Answer from the drawing. Dimensions are ordinates in mm from the lowest x, y and z of the part. A direction names the side the tool comes from. Give positions to 0.01 mm unless a question says otherwise; leave off trailing zeros. Loops run counter-clockwise (first coordinate to the right, second up) from the corner with the lowest first, then second, coordinate; pieces in that order, holes last. Notation, with made-up numbers: (72, 23) - (101, 23) arc R36 cw to (101, 60) - close; hole circle Ø9 at (65.25, 29.5). An arc over 180 degrees is marked (long way). One line per question, with ' | ' between items. Start each with the question number.
1. Which of the six approach directions +Z, -Z, +X, -X, +Y, -Y give full straight-line access (tool end or side, diameter ignored) to the marked faces 3 and 4?
2. Section C-C (z = 2.1) is taken. Determine the outline of the cut face in (x, y).
3. For a pull along Y with two mould halves and no side action, classify the marked faces 1 and 2 as released by +Y, released by -Y, zero draft, split by the parting line, or undercut.
4. Section A-A (y = 6.4) is taken. Determine the outline of the cut face in (x, z), plus the area to 3 significant figures.
5. Find the intervals of material crossed by line 1 (Y direction, x = 6.4, z = 0.35); line 2 (Y direction, x = 6.4, z = 1.85); line 3 (X direction, y = 6, z = 0.75), in increasing order.
6. Section D-D (z = 1.05) is taken. Determine the outline of the cut face in (x, y), plus the area to 3 significant figures.
7. Each of these flat-tipped pins is pushed along its axis until it touches: pin 1 (1 mm diameter, centred on x = 11.5, z = 1.5, fed in from +Y); pin 2 (1.4 mm diameter, centred on x = 6.4, y = 6.4, fed in from -Z). Where does it stop, or does it pass through?
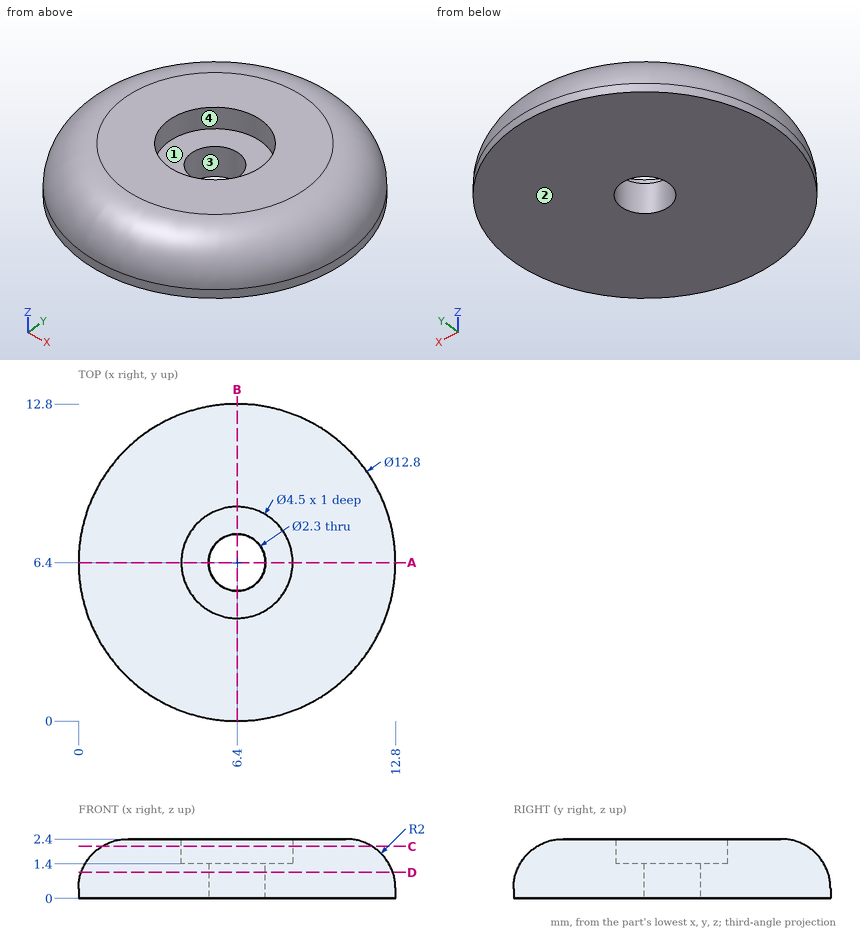
Conclusion:
1) face 3: +Z, -Z | face 4: +Z
2) outline: circle Ø10.91 at (6.4, 6.4); hole circle Ø4.5 at (6.4, 6.4)
3) face 1: undercut | face 2: zero draft
4) outline: (0, 0) - (5.25, 0) - (5.25, 1.4) - (4.15, 1.4) - (4.15, 2.4) - (2, 2.4) arc R2 ccw to (0, 0.4) - close; (7.55, 0) - (12.8, 0) - (12.8, 0.4) arc R2 ccw to (10.8, 2.4) - (8.65, 2.4) - (8.65, 1.4) - (7.55, 1.4) - close | area: 21.3 mm²
5) line 1: 0 to 5.25, 7.55 to 12.8 | line 2: 0.62 to 4.15, 8.65 to 12.18 | line 3: 0.04 to 5.32, 7.48 to 12.76
6) outline: circle Ø12.58 at (6.4, 6.4); hole circle Ø2.3 at (6.4, 6.4) | area: 120 mm²
7) pin 1: y = 10.5 | pin 2: through
